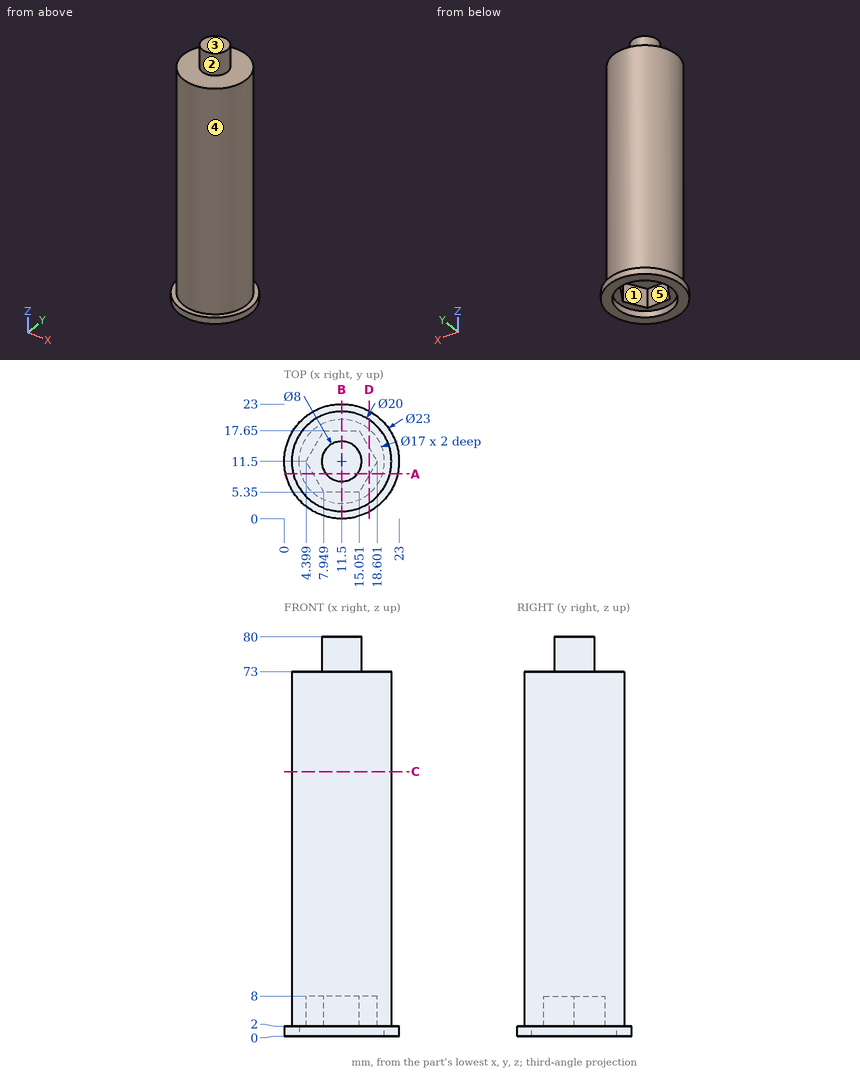
Study the drawing (mm; zero at the part's minimum x, y, z) and answer. A direction names the side the tool comes from. Give positions to 0.01 mm unless a question says otherwise; leave off trailing zeros. Order: outer loops, then holes, each group sorted by start corner. A loop starts at its lowest first (then second) coordinate and runs counter-clockwise, first axis right, second up.
1) Find section A-A on y = 9. Write down the section's boundary in (x, z) (1 decimal).
Reported:
outline: (0.3, 0) - (3.4, 0) - (3.4, 2) - (5.8, 2) - (5.8, 8) - (17.2, 8) - (17.2, 2) - (19.6, 2) - (19.6, 0) - (22.7, 0) - (22.7, 2) - (21.2, 2) - (21.2, 73) - (14.6, 73) - (14.6, 80) - (8.4, 80) - (8.4, 73) - (1.8, 73) - (1.8, 2) - (0.3, 2) - close
2) For the marked faces 1 and 2, determine the directions among +Z, -Z, +X, -X, +Y, -Y from which every point of the face is accessible in a straight line to the end or side of a thin tool.
Reported:
face 1: -Z
face 2: +Z
3) Find section B-B on x = 11.5. Write down the section's boundary in (y, z), then the cut area to 3 significant figures.
Reported:
outline: (0, 0) - (3, 0) - (3, 2) - (5.35, 2) - (5.35, 8) - (17.65, 8) - (17.65, 2) - (20, 2) - (20, 0) - (23, 0) - (23, 2) - (21.5, 2) - (21.5, 73) - (15.5, 73) - (15.5, 80) - (7.5, 80) - (7.5, 73) - (1.5, 73) - (1.5, 2) - (0, 2) - close
area: 1,410 mm2
4) Determine the mould class of the marked faces 3, 4 and 5 for opening direction Y: pulls with the +Y half, pulls with the -Y half, needs draft (parallel to the pull), parting line crosses it, or undercut.
Reported:
face 3: needs draft
face 4: parting line crosses it
face 5: undercut
5) Find section C-C on z = 53. Write down the section's boundary in (x, y).
Reported:
outline: circle Ø20 at (11.5, 11.5)
6) Find section D-D on x = 17. Write down the section's boundary in (y, z), then the cut area to 3 significant figures.
Reported:
outline: (1.4, 0) - (5.02, 0) - (5.02, 2) - (8.73, 2) - (8.73, 8) - (14.27, 8) - (14.27, 2) - (17.98, 2) - (17.98, 0) - (21.6, 0) - (21.6, 2) - (19.85, 2) - (19.85, 73) - (3.15, 73) - (3.15, 2) - (1.4, 2) - close
area: 1,170 mm2
7) Consider line 1 along Y through (x, z) = (11.5, 0.5); line 2 along Z through (x, y) = (9.75, 16.25); line 3 along Z through (x, y) = (11.75, 14.75). Determine where each line is inside the solid, lowest interval first.
Reported:
line 1: y = 0 to 3, 20 to 23
line 2: z = 8 to 73
line 3: z = 8 to 80
8) Given P1, Ø12, axis at y = 4.5, z = 60.5, coming from the +X side; P2, Ø3, axis at x = 10, z = 5.5, coming from the +Y side; P3, Ø2, axis at y = 7.5, z = 54, coming from the -X side, each flat-ended and moving along its own axis, determine where each tip first touches the part or whether it passes through.
Reported:
P1: stops at x = 21.45
P2: stops at y = 21.5
P3: stops at x = 1.96
